Build history of the part. All positions in model axes, mm. Give positions to 0.01 mm unless a question says otherwise; leave off trailing zeros. Order: outer loops, then holes, each group sorted by start corner. A loop starts at its lowest first (then second) coordinate and runs counter-clockwise, first axis right, second up. Notation, with made-up numbers: (0, 26.5) - (29, 26.5) arc R32 cw to (29, 54.5) - close; hole circle Ø2 at (-10, 19.25). An arc over 180 degrees is marked (long way). Write each question's results on one line, items separated by ' | '. Start each with the question number.
1) Drop flat-ended pins along their axis: pin 1 Ø2 at (x, z) = (-7.5, -23.5) entering from +Y; pin 2 Ø3 at (x, z) = (3, 37.5) entering from -Y; pin 3 Ø0.9 at (y, z) = (2.5, 50) entering from -X. Give the stop position or say it passes through.
2) Cut at C-C on z = -13. List the corners of the cut face in (x, y), plus the area to 3 significant figures.
3) Cut at B-B on x = 0. List the corners of the cut face in (y, z), plus the area to 3 significant figures.
4) Two-plate mould, pull along X, no slides. Class faces 1 (the face through (0, 0, -35)), 2 (the face through (0, 2, 45)), 3 (the face through (0, -3, 45)): +X half, -X half, draft (parallel to the pull), parting line (faces both ways), or undercut.
5) Cut at D-D on z = 45.5. List the corners of the cut face in (x, y).
6) Drill centre lines: line 1 along Z through (x, y) = (8.5, -8.5); line 2 along X through (y, z) = (-11.5, -23); line 3 along X through (y, z) = (15, 29). Where is each one in solid material? Low to high. Write a range as from..to.
7) Cut at A-A on y = 0. List the corners of the cut face in (x, z), plus the area to 3 significant figures.
from build123d import *

# Parameters (mm, degrees)
SKETCH_1_R      = 18.5
EXTRUDE_1_DEPTH = 35
EXTRUDE_2_DEPTH = 20


with BuildPart() as part:
    # 草图1 → 凸台-拉伸1 (new, symmetric)
    with BuildSketch(Plane.XY):
        Circle(SKETCH_1_R)
    extrude(amount=EXTRUDE_1_DEPTH, both=True)

    # 草图2 → 凸台-拉伸2 (add)
    with BuildSketch(Plane.XY.offset(35)):
        with BuildLine():
            Line((-1, 2.828427125), (-1, 2))
            Line((-1, 2), (1, 2))
            Line((1, 2), (1, 2.828427125))
            ThreePointArc((1, 2.828427125), (0, -3), (-1, 2.828427125))
        make_face()
    extrude(amount=EXTRUDE_2_DEPTH)


solid = part.part
Results:
1) pin 1: y = 17.32 | pin 2: y = -2.6 | pin 3: x = -2.19
2) outline: circle Ø37 at (0, 0) | area: 1,080 mm^2
3) outline: (-18.5, -35) - (18.5, -35) - (18.5, 35) - (2, 35) - (2, 55) - (-3, 55) - (-3, 35) - (-18.5, 35) - close | area: 2,690 mm^2
4) face 1: draft | face 2: undercut | face 3: parting line
5) outline: (-1, 2) - (-1, 2.83) arc R3 ccw (long way) to (1, 2.83) - (1, 2) - close
6) line 1: -35..35 | line 2: -14.49..14.49 | line 3: -10.83..10.83
7) outline: (-18.5, -35) - (18.5, -35) - (18.5, 35) - (3, 35) - (3, 55) - (-3, 55) - (-3, 35) - (-18.5, 35) - close | area: 2,710 mm^2
